```python
from build123d import *

# Parameters (mm, degrees)
F0_R     = 12.5
F0_R_2   = 5
F3_DEPTH = 25
F1_SIZE  = 0.5
F2_SIZE  = 1


with BuildPart() as f3:
    # F0 (on Front) → F3 (new body)
    with BuildSketch(Plane.XZ):
        with BuildLine():
            ThreePointArc((5.75, -16.528385), (14.263152, -10.13965), (17.5, 0))
            ThreePointArc((17.5, 0), (14.263152, 10.13965), (5.75, 16.528385))
            ThreePointArc((5.75, 16.528385), (-17.5, 0), (5.75, -16.528385))
        make_face()
        Circle(F0_R, mode=Mode.SUBTRACT)
        with BuildLine():
            ThreePointArc((5.75, 16.528385), (14.263152, 10.13965), (17.5, 0))
            ThreePointArc((17.5, 0), (14.263152, -10.13965), (5.75, -16.528385))
            Line((5.75, -16.528385), (36.971429, -5.666875))
            ThreePointArc((36.971429, -5.666875), (29, 0), (36.971429, 5.666875))
            Line((36.971429, 5.666875), (5.75, 16.528385))
        make_face()
        with BuildLine():
            ThreePointArc((41, 0), (39.890223, 3.476451), (36.971429, 5.666875))
            ThreePointArc((36.971429, 5.666875), (29, 0), (36.971429, -5.666875))
            ThreePointArc((36.971429, -5.666875), (39.890223, -3.476451), (41, 0))
        make_face()
        with Locations((35, 0)):
            Circle(F0_R_2, mode=Mode.SUBTRACT)
    extrude(amount=F3_DEPTH)

    # F1
    f1_edges = [f3.edges().sort_by_distance(p)[0] for p in [
        (-12.5, -25, 0),
    ]]
    chamfer(f1_edges, length=F1_SIZE)

    # F2
    f2_edges = [f3.edges().sort_by_distance(p)[0] for p in [
        (-12.5, 0, 0),
    ]]
    chamfer(f2_edges, length=F2_SIZE)


solid = f3.part
```
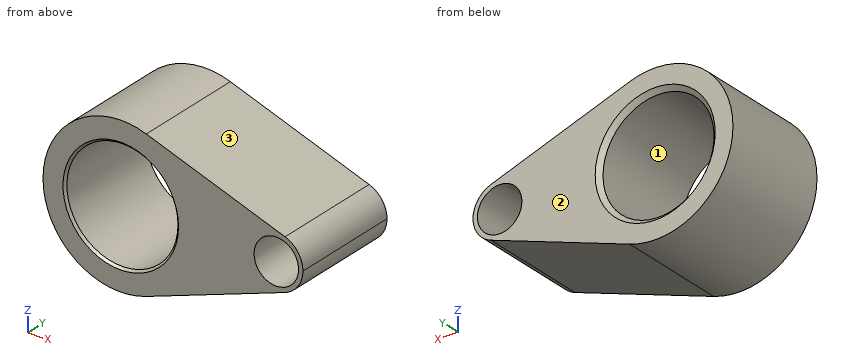
Can you work these out from the model? Positions are in its coordinate system, mm. Face numbers are marked on the shaded views. Coordinates: 2 decimals unless noted, no trailing zeros. Loops run counter-clockwise (first coordinate to the right, second up) from the corner with the lowest first, then second, coordinate; pieces in that order, holes last. Notation, with made-up numbers: M 87.25,85.25 L 144.25,85.25 A6 ccw 144.25,96.25 Z; hole C 49.5,-4.75 d4. An arc over 180 degrees is marked long. Put each result on its own line as item: value. Start each with the question number.
(1) I need wall thicknesses on probe 1 along Z at (x, y) = (0, -10); probe 2 along X at (y, z) = (-21, -4); probe 3 along Z at (x, y) = (38.5, -18.25). Which ranges of each line are inside material? Lowest first, please.
(2) Will these pins go through, and if not, where does the flat tip stop? pin 1 Ø1 at (y, z) = (-15, -7.5) entering from -X; pin 2 Ø2 at (x, y) = (14, -12) entering from -Z; pin 3 Ø5 at (x, y) = (19, -19.5) entering from -Z.
(3) Imagine slicing it at B-B on x = 0. List the corners of the cut face in (y, z) for me, and give its area (3 significant figures).
(4) Imagine slicing it at D-D on x = 20. List the corners of the cut face in (y, z) for me.
(5) Imagine slicing it at C-C on x = 35. List the corners of the cut face in (y, z) for me.
(6) Imagine slicing it at A-A on y = -9. List the corners of the cut face in (x, z) for me, and give its area (3 significant figures).
(7) We'd pull the mould along Z, two halves only. Please class the marked faces 1, 2 and 3: +Z half, -Z half, draft (parallel to the pull), parting line (faces both ways), or undercut.
Worked answers:
1. probe 1: z = -17.5 to -12.5, 12.5 to 17.5
1. probe 2: x = -17.04 to -11.84, 11.84 to 32, 38 to 39.47
1. probe 3: z = -4.87 to -3.57, 3.57 to 4.87
2. pin 1: stops at x = -16.04
2. pin 2: stops at z = -14.01
2. pin 3: stops at z = -12.79
3. outline: M -25,-17.5 L 0,-17.5 L 0,-13.5 L -1,-12.5 L -24.5,-12.5 L -25,-13 Z; M -25,13 L -24.5,12.5 L -1,12.5 L 0,13.5 L 0,17.5 L -25,17.5 Z
3. area: 249 mm2
4. outline: M -25,-11.57 L 0,-11.57 L 0,11.57 L -25,11.57 Z
5. outline: M -25,-6.35 L 0,-6.35 L 0,-5 L -25,-5 Z; M -25,5 L 0,5 L 0,6.35 L -25,6.35 Z
6. outline: M 5.75,-16.53 L 36.97,-5.67 A6 ccw 41,0 A6 ccw 36.97,5.67 L 5.75,16.53 A17.5 ccw long Z; hole C 0,0 d25; hole C 35,0 d10
6. area: 836 mm2
7. face 1: undercut
7. face 2: draft
7. face 3: +Z half
